For this review, use the dimensioned drawing (mm, ordinates from the lowest corner) and the shaded views. Round coordinates to 2 decimals unless told otherwise and drop trailing zeros. Order: outer loops, then holes, each group sorted by start corner. A loop starts at its lowest first (then second) coordinate and runs counter-clockwise, first axis right, second up. Notation, with made-up numbers: M -36.75,62.25 L 7.25,62.25 A13 cw 7.25,70.25 Z; hole C -18,2 d4. An arc over 180 degrees is marked long. Answer as CSV lines item,"result". Start each with the question number.
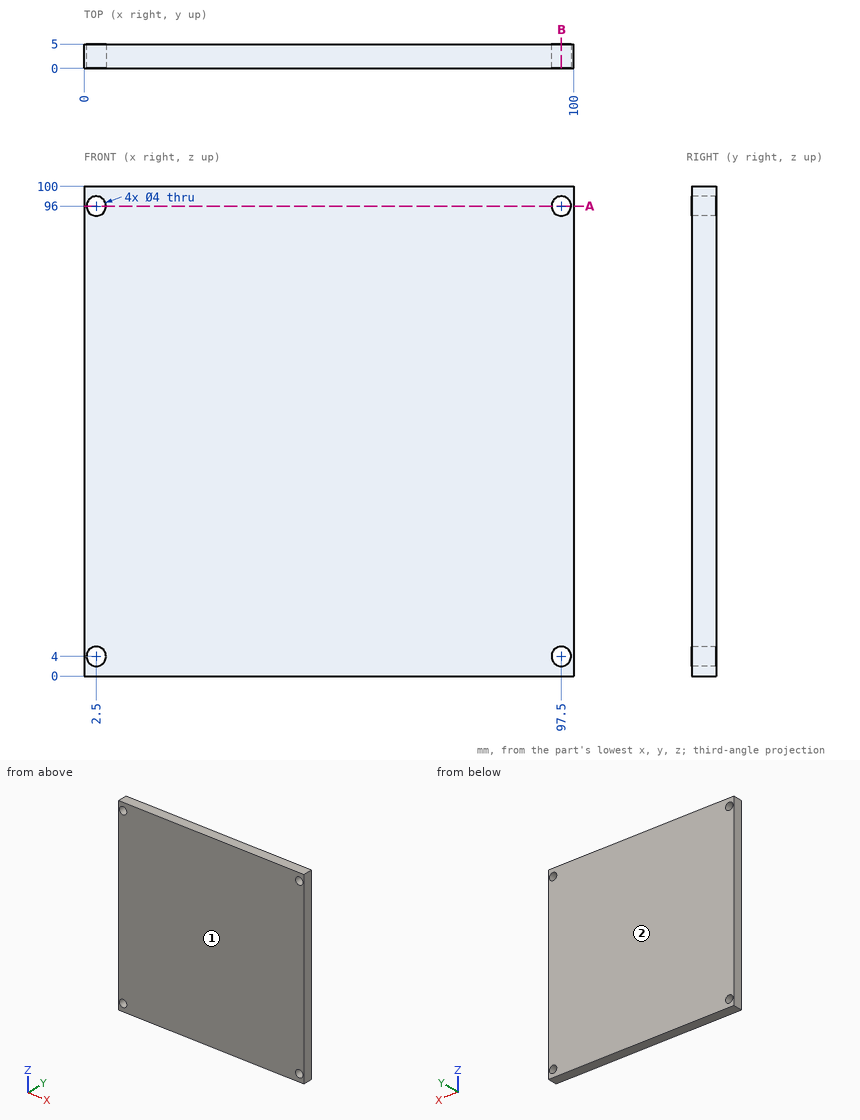
Item 1: For pin 1 (2.5 mm diameter, centred on x = 97.5, z = 4, fed in from -Y), flat-tipped, find the tip position at first contact; note if it passes through.
Item 2: Consider section A-A (z = 96). State the section outline as (x, y) points.
Item 3: Consider section B-B (x = 97.5). State the section outline as (y, z) points, and give its area (3 significant figures).
Item 4: The part is to be moulded in two halves that separate along Y. For the marked faces 1 and 2, say which applies: +Y half, -Y half, draft (parallel to the pull), parting line (faces both ways), or undercut.
Item 5: Wall thickness on probe 1 along X at (y, z) = (2.8, 4); probe 2 along Z at (x, y) = (97.5, 3.6); probe 3 along X at (y, z) = (3.5, 94.5): over which ranges is each line inside the solid? List them lowest first. Write a range as [from, to].
Reported:
1,pin 1,"passes through"
2,outline,"M 0,0 L 0.5,0 L 0.5,5 L 0,5 Z; M 4.5,0 L 95.5,0 L 95.5,5 L 4.5,5 Z; M 99.5,0 L 100,0 L 100,5 L 99.5,5 Z"
3,outline,"M 0,0 L 5,0 L 5,2 L 0,2 Z; M 0,6 L 5,6 L 5,94 L 0,94 Z; M 0,98 L 5,98 L 5,100 L 0,100 Z"
3,area,"460 mm²"
4,face 1,"-Y half"
4,face 2,"+Y half"
5,probe 1,"x = [0, 0.5], [4.5, 95.5], [99.5, 100]"
5,probe 2,"z = [0, 2], [6, 94], [98, 100]"
5,probe 3,"x = [0, 1.18], [3.82, 96.18], [98.82, 100]"
